Here's how the part is built. I have some questions about the finished solid (model axes, mm). Coordinates: 2 decimals unless noted, no trailing zeros. Order: outer loops, then holes, each group sorted by start corner. A loop starts at its lowest first (then second) coordinate and runs counter-clockwise, first axis right, second up.
```python
from build123d import *

# Parameters (mm, degrees)
SKETCH_1_W          = 105
SKETCH_1_H          = 75
SKETCH_1_R          = 2
EXTRUDE_1_DEPTH     = 3
FILLET_1_R          = 2
SKETCH_2_R          = 2.5
CUT_EXTRUDE_1_DEPTH = 10


with BuildPart() as part:
    # 스케치1 → 보스-돌출1 (new body)
    with BuildSketch(Plane(origin=(0, 0, 0), x_dir=(1, 0, 0), z_dir=(0, 1, 0))):
        Rectangle(SKETCH_1_W, SKETCH_1_H)
        with Locations(Location((-48, 33, 0), (0, 0, 270))):
            Circle(SKETCH_1_R, mode=Mode.SUBTRACT)
        with Locations(Location((-48, -33, 0), (0, 0, 270))):
            Circle(SKETCH_1_R, mode=Mode.SUBTRACT)
        with Locations(Location((48, -33, 0), (0, 0, 270))):
            Circle(SKETCH_1_R, mode=Mode.SUBTRACT)
        with Locations(Location((48, 33, 0), (0, 0, 270))):
            Circle(SKETCH_1_R, mode=Mode.SUBTRACT)
    extrude(amount=EXTRUDE_1_DEPTH)

    # 필렛1
    fillet_1_edges = [part.edges().sort_by_distance(p)[0] for p in [
        (52.5, 1.5, 37.5),
        (-52.5, 1.5, 37.5),
        (-52.5, 1.5, -37.5),
        (52.5, 1.5, -37.5),
    ]]
    fillet(fillet_1_edges, radius=FILLET_1_R)

    # 스케치2 → 컷-돌출1 (cut)
    with BuildSketch(Plane(origin=(0, 3, 0), x_dir=(1, 0, 0), z_dir=(0, 1, 0))):
        with Locations(Location((-37.5, -22.5, 0), (0, 0, 270))):
            Circle(SKETCH_2_R)
        with Locations(Location((37.5, -22.5, 0), (0, 0, 270))):
            Circle(SKETCH_2_R)
        with Locations(Location((37.5, 22.5, 0), (0, 0, 270))):
            Circle(SKETCH_2_R)
        with Locations(Location((-37.5, 22.5, 0), (0, 0, 270))):
            Circle(SKETCH_2_R)
    extrude(amount=-CUT_EXTRUDE_1_DEPTH, mode=Mode.SUBTRACT)


solid = part.part
```
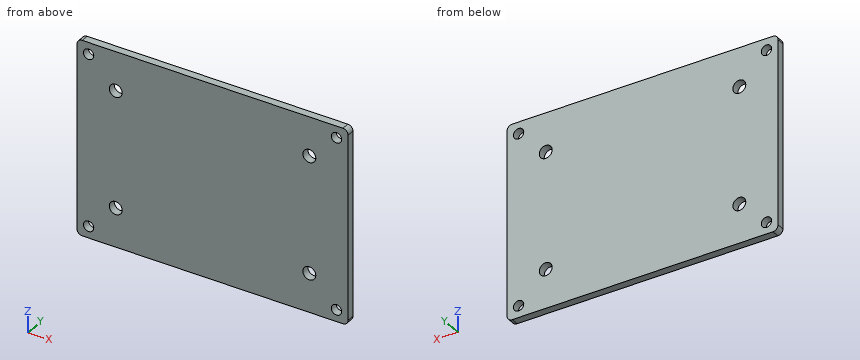
Q1. Will this pin go through, and if not, where does the flat tip stop? pin 1 (3.5 mm diameter, centred on x = 48, z = 33, fed in from -Y).
Q2. If we section it at C-C on y = 1.6: Give the number of separate pieces and of enclosed holes in the cut face, then the cut area to 3 significant figures.
Q3. I need wall thicknesses on L1, parallel to X at y = 1.2, z = 33; L2, parallel to X at y = 1.15, z = 22.5; L3, parallel to Z at x = -35.5, y = 0.3. Which ranges of each line are inside material? Lowest first, please.
Q4. If we section it at A-A on x = 48: Write out the boundary of the cut face in (y, z), then the cut area to 3 significant figures.
Q5. If we section it at B-B on z = 33: Write out the boundary of the cut face in (x, y), then the cut area to 3 significant figures.
Reply:
1. pin 1: passes through
2. separate pieces: 1
2. enclosed holes: 8
2. area: 7,740 mm2
3. L1: x = -52.5 to -50, -46 to 46, 50 to 52.5
3. L2: x = -52.5 to -40, -35 to 35, 40 to 52.5
3. L3: z = -37.5 to -24, -21 to 21, 24 to 37.5
4. outline: (0, -37.5) - (3, -37.5) - (3, -35) - (0, -35) - close; (0, -31) - (3, -31) - (3, 31) - (0, 31) - close; (0, 35) - (3, 35) - (3, 37.5) - (0, 37.5) - close
4. area: 201 mm2
5. outline: (-52.5, 0) - (-50, 0) - (-50, 3) - (-52.5, 3) - close; (-46, 0) - (46, 0) - (46, 3) - (-46, 3) - close; (50, 0) - (52.5, 0) - (52.5, 3) - (50, 3) - close
5. area: 291 mm2
